Read the model definition and answer for the solid it produces. Units are mm, in the model's axes. A direction names the side the tool comes from. Give positions to 0.01 mm unless a question says otherwise; leave off trailing zeros. Order: outer loops, then holes, each group sorted by start corner. A loop starts at its lowest first (then second) coordinate and runs counter-clockwise, first axis right, second up. Notation, with made-up numbers: (5, 58.5) - (19, 58.5) arc R27 ccw to (19, 76.5) - close; hole circle Ø9 at (89.5, 85.25). An arc over 180 degrees is marked (long way). Write each question's results on one line, items separated by ' | '. Start each with the question number.
Q1. Find section D-D on y = 5. Give the vertices of the cut face in (x, z).
Q2. Find the intervals of material crossed by line 1 along Y through (x, z) = (31, 1.65); line 2 along Y through (x, z) = (25, 2.1); line 3 along X through (y, z) = (-26.5, 2.2), in increasing order. Write a range as from..to.
Q3. A tool of negligible diameter and unlimited length cuts with its end or side. For faces 4 (the face through (40.04, -0.11, 1.52)), 5 (the face through (19.7, 0.4, 0)), from which of +Z, -Z, +X, -X, +Y, -Y can it reach the whole face along a straight path? Write none if from no direction.
Q4. Find section B-B on y = -32.5. Give the vertices of the cut face in (x, z), and give its area (3 significant figures).
Q5. A flat-ended cylindrical pin translates along its axis: P1, Ø10, axis at x = 3.5, y = -7, coming from the -Z side. Find the tip coordinate at first contact, or state that the pin passes through.
Q6. Find section C-C on x = 9. Give the vertices of the cut face in (y, z).
Q7. For a pull along X with two mould halves and no side action, classify faces 1 (the face through (32.339, 4.445, 1.521)), 2 (the face through (69.42, -9.08, 1.48)), 3 (the face through (19.7, 0.4, 3)) as +X half, -X half, draft (parallel to the pull), parting line (faces both ways), or undercut.
Q8. Find section A-A on z = 2.3. Give the vertices of the cut face in (x, y).
from build123d import *

# Parameters (mm, degrees)
EXTRUDE_1_DEPTH     = 3
SKETCH_3_R          = 1.45
CUT_EXTRUDE_2_DEPTH = 93.952945085
FILLET_1_R          = 10


with BuildPart() as part:
    # 草图1 → 凸台-拉伸1 (new body)
    with BuildSketch(Plane.XY):
        with BuildLine():
            Line((-45, -37.5), (-37, -37.5))
            ThreePointArc((-37, -37.5), (-23.489142232, -13.827379664), (0, 0))
            Line((0, 0), (40, 0))
            ThreePointArc((40, 0), (63.489142232, -13.827379664), (77, -37.5))
            Line((77, -37.5), (85, -37.5))
            ThreePointArc((85, -37.5), (68.488362784, -8.076814205), (40, 10))
            Line((40, 10), (0, 10))
            ThreePointArc((0, 10), (-28.488362784, -8.076814205), (-45, -37.5))
        make_face()
    extrude(amount=EXTRUDE_1_DEPTH)

    # 草图3 → 切除-拉伸2 (cut, through all)
    with BuildSketch(Plane.XY.offset(3)):
        with Locations((9, 5)):
            Circle(SKETCH_3_R)
        with Locations((31, 5)):
            Circle(SKETCH_3_R)
    extrude(amount=-CUT_EXTRUDE_2_DEPTH, mode=Mode.SUBTRACT)

    # 圆角1
    fillet_1_edges = [part.edges().sort_by_distance(p)[0] for p in [
        (0, 10, 1.5),
        (40, 10, 1.5),
        (40, 0, 1.5),
        (0, 0, 1.5),
    ]]
    fillet(fillet_1_edges, radius=FILLET_1_R)


solid = part.part
Working result:
1) outline: (-11.52, 0) - (7.55, 0) - (7.55, 3) - (-11.52, 3) - close; (10.45, 0) - (29.55, 0) - (29.55, 3) - (10.45, 3) - close; (32.45, 0) - (51.52, 0) - (51.52, 3) - (32.45, 3) - close
2) line 1: 0..3.55, 6.45..10 | line 2: 0..10 | line 3: -40.99..-32.73, 72.73..80.99
3) face 4: +Z, -Z, -Y | face 5: -Z, +X, -X, +Y, -Y
4) outline: (-43.44, 0) - (-35.41, 0) - (-35.41, 3) - (-43.44, 3) - close; (75.41, 0) - (83.44, 0) - (83.44, 3) - (75.41, 3) - close | area: 48.2 mm²
5) P1: through
6) outline: (0, 0) - (3.55, 0) - (3.55, 3) - (0, 3) - close; (6.45, 0) - (10, 0) - (10, 3) - (6.45, 3) - close
7) face 1: undercut | face 2: +X half | face 3: draft
8) outline: (-45, -37.5) - (-37, -37.5) arc R53 cw to (-1.53, -0.45) arc R10 cw to (1.44, 0) - (38.56, 0) arc R10 cw to (41.53, -0.45) arc R53 cw to (77, -37.5) - (85, -37.5) arc R69 ccw to (41.71, 9.41) arc R10 ccw to (38.33, 10) - (1.67, 10) arc R10 ccw to (-1.71, 9.41) arc R69 ccw to start; hole circle Ø2.9 at (9, 5); hole circle Ø2.9 at (31, 5)
